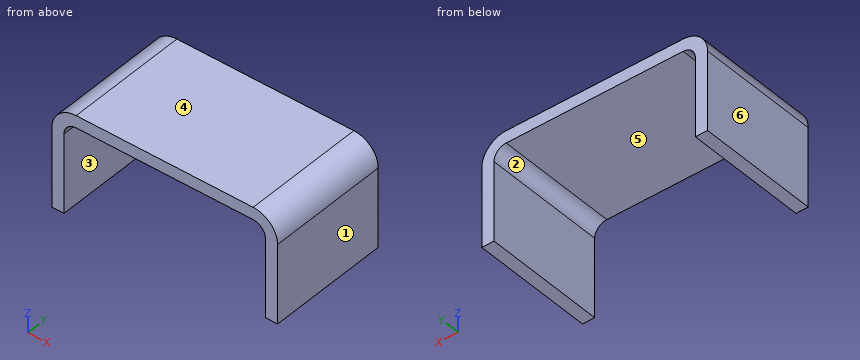
from build123d import *

# Parameters (mm, degrees)
BOSS_EXTRUDE2_DEPTH = 20


with BuildPart() as part:
    # Sketch1 → Boss-Extrude2 (new body)
    with BuildSketch(Plane(origin=(0, 0, 0), x_dir=(1, 0, 0), z_dir=(0, 1, 0))):
        with BuildLine():
            Line((1.36644496, -14.394460771), (-13.63355504, -14.394460771))
            ThreePointArc((-13.63355504, -14.394460771), (-15.047768603, -13.808674334), (-15.63355504, -12.394460771))
            Line((-15.63355504, -12.394460771), (-15.63355504, 0.505539229))
            Line((-15.63355504, 0.505539229), (-17.63355504, 0.505539229))
            Line((-17.63355504, 0.505539229), (-17.63355504, -12.394460771))
            ThreePointArc((-17.63355504, -12.394460771), (-16.461982165, -15.222887896), (-13.63355504, -16.394460771))
            Line((-13.63355504, -16.394460771), (1.36644496, -16.394460771))
            Line((1.36644496, -16.394460771), (15.36644496, -16.394460771))
            ThreePointArc((15.36644496, -16.394460771), (18.194872084, -15.222887896), (19.36644496, -12.394460771))
            Line((19.36644496, -12.394460771), (19.36644496, 0.505539229))
            Line((19.36644496, 0.505539229), (17.36644496, 0.505539229))
            Line((17.36644496, 0.505539229), (17.36644496, -12.394460771))
            ThreePointArc((17.36644496, -12.394460771), (16.780658522, -13.808674334), (15.36644496, -14.394460771))
            Line((15.36644496, -14.394460771), (1.36644496, -14.394460771))
        make_face()
    extrude(amount=BOSS_EXTRUDE2_DEPTH)


solid = part.part
The model under review builds one solid part; all positions refer to its coordinate system, in mm. Face numbers are marked on the shaded views. A direction names the side the tool comes from. Coordinates: 2 decimals unless noted, no trailing zeros. Loops run counter-clockwise (first coordinate to the right, second up) from the corner with the lowest first, then second, coordinate; pieces in that order, holes last.
(1) Draft analysis for pull direction X (two halves, no side actions). For the marked faces 1, 2, 3 and 4, state which applies: +X half, -X half, draft (parallel to the pull), parting line (faces both ways), or undercut.
Determined:
face 1: +X half
face 2: undercut
face 3: undercut
face 4: draft
(2) Consider section A-A, the plane z = 3.75. Give the boundary of the cut face in (x, y), plus the area to 3 significant figures.
Determined:
outline: (-17.63, 0) - (-15.63, 0) - (-15.63, 20) - (-17.63, 20) - close; (17.37, 0) - (19.37, 0) - (19.37, 20) - (17.37, 20) - close
area: 80.0 mm2
(3) Insertion check: P1, Ø4, axis at x = -10, y = 14.5, coming from the -Z side; P2, Ø1.5, axis at y = 6.5, z = 14.5, coming from the +X side. Each pin has a flat end and moves straight along its axis. Give the tip position at first contact, or say it passes through.
Determined:
P1: stops at z = 14.39
P2: stops at x = 19.13
(4) Wall thickness on L1, parallel to X at y = 15, z = 12; L2, parallel to Z at x = 7.5, y = 10.75; L3, parallel to X at y = 13.5, z = 12.75: over which ranges is each line inside the solid? List them lowest first.
Determined:
L1: x = -17.63 to -15.63, 17.37 to 19.37
L2: z = 14.39 to 16.39
L3: x = -17.62 to -15.6, 17.33 to 19.35
(5) Tool access review of the marked faces 5 and 6: name each direction out of +Z, -Z, +X, -X, +Y, -Y from which nothing blocks a thin tool from reaching the whole face with its end or side.
Determined:
face 5: -Z, +Y, -Y
face 6: +Z, -Z, -X, +Y, -Y
(6) Consider section B-B, the plane y = 14.5. Give the boundary of the cut face in (x, z).
Determined:
outline: (-17.63, -0.51) - (-15.63, -0.51) - (-15.63, 12.39) arc R2 cw to (-13.63, 14.39) - (15.37, 14.39) arc R2 cw to (17.37, 12.39) - (17.37, -0.51) - (19.37, -0.51) - (19.37, 12.39) arc R4 ccw to (15.37, 16.39) - (-13.63, 16.39) arc R4 ccw to (-17.63, 12.39) - close
(7) Consider section D-D, the plane z = 15.25. Give the boundary of the cut face in (x, y).
Determined:
outline: (-16.43, 0) - (18.17, 0) - (18.17, 20) - (-16.43, 20) - close
(8) Consider section C-C, the plane x = 11.5. Give the boundary of the cut face in (y, z), plus the area to 3 significant figures.
Determined:
outline: (0, 14.39) - (20, 14.39) - (20, 16.39) - (0, 16.39) - close
area: 40.0 mm2
